The figure shows three views and two pictorial views of one solid part (mm, origin at its lowest corner). Answer the questions. A direction names the side the tool comes from. Round coordinates to 2 decimals unless told otherwise and drop trailing zeros. Order: outer loops, then holes, each group sorted by start corner. A loop starts at its lowest first (then second) coordinate and runs counter-clockwise, first axis right, second up. Notation, with made-up numbers: (54.25, 15) -> (87.25, 15) arc R24 ccw to (87.25, 48) -> close; hole circle Ø9 at (79, 0.5). An arc over 180 degrees is marked (long way). Answer as a JSON object with one key per item and string values. Group by question number.
Item 1: The mould has two halves that part along Z. Classify the marked faces 3, 4 and 5: pulls with the +Z half, pulls with the -Z half, needs draft (parallel to the pull), parting line crosses it, or undercut.
Item 2: Section B-B, the plane y = 7.5 is taken. Write down the section's boundary in (x, z) (1 decimal).
Item 3: Given P1, Ø4, axis at x = 38, y = 9.5, coming from the -Z side; P2, Ø10, axis at y = 6, z = 99.5, coming from the +X side (1 decimal); P3, Ø10, axis at x = 16.5, z = 29, coming from the +Y side (1 decimal), each flat-ended and moving along its own axis, determine where each tip first touches the part or whether it passes through.
Item 4: Section A-A, the plane y = 27 is taken. Write down the section's boundary in (x, z), plus the area to 3 significant figures.
Item 5: Section C-C, the plane z = 10.5 is taken. Write down the section's boundary in (x, y) (1 decimal), plus the area to 3 significant figures.
Item 6: Consider probe 1 along Z at (x, y) = (55, 29) (1 decimal); probe 2 along X at (y, z) = (30.5, 67) (1 decimal); probe 3 along Y at (x, z) = (105.5, 46) (1 decimal). Determine where each line is inside the solid, lowest interval first. Write a range as from..to.
Item 7: For the marked faces 1 and 2, determine the directions among +Z, -Z, +X, -X, +Y, -Y from which every point of the face is accessible in a straight line to the end or side of a thin tool.
Item 8: Section D-D, the plane x = 98 is taken. Write down the section's boundary in (y, z) (1 decimal).
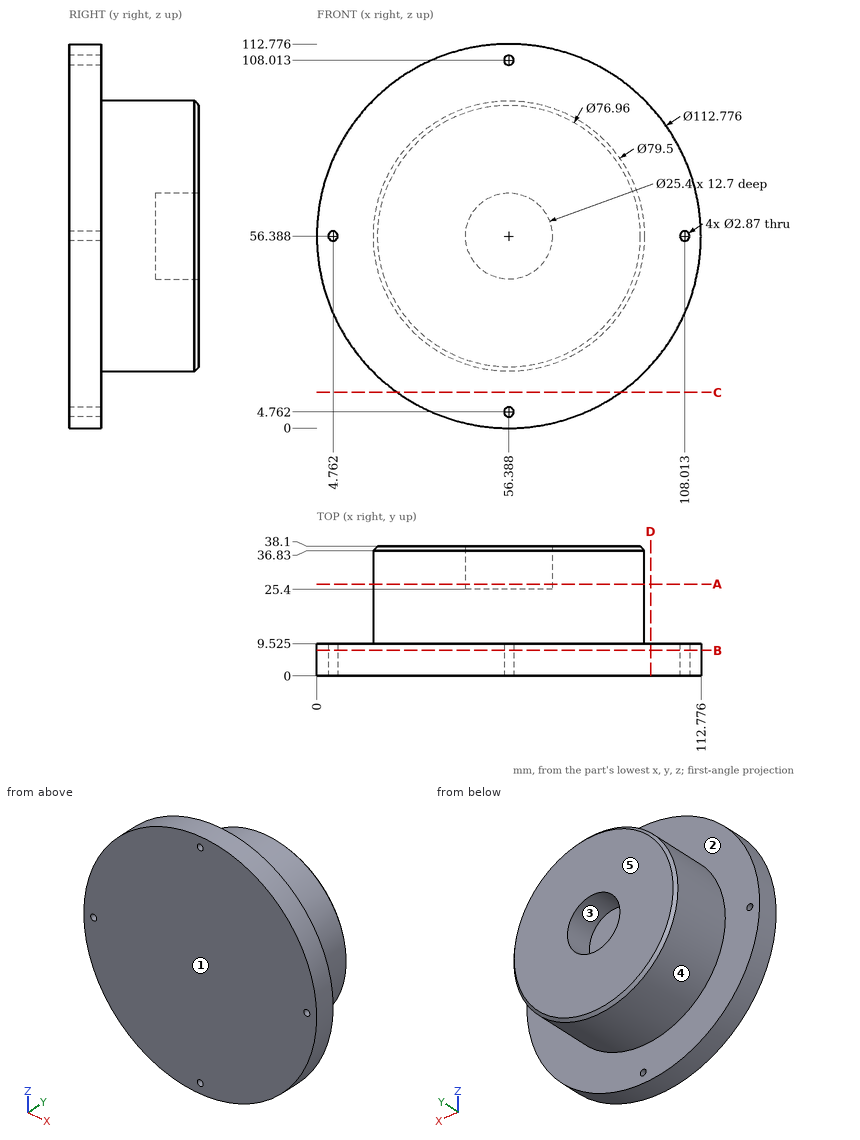
Values found:
{
 "1": {"face 3": "undercut", "face 4": "parting line crosses it", "face 5": "needs draft"},
 "2": {"outline": "circle Ø112.8 at (56.4, 56.4); hole circle Ø2.9 at (4.8, 56.4); hole circle Ø2.9 at (56.4, 4.8); hole circle Ø2.9 at (56.4, 108); hole circle Ø2.9 at (108, 56.4)"},
 "3": {"P1": "z = 2.43", "P2": "x = 97.9", "P3": "y = 9.5"},
 "4": {"outline": "circle Ø79.5 at (56.39, 56.39); hole circle Ø25.4 at (56.39, 56.39)", "area": "4,460 mm2"},
 "5": {"outline": "(23.6, 0) -> (89.2, 0) -> (89.2, 9.5) -> (23.6, 9.5) -> close", "area": "624 mm2"},
 "6": {"probe 1": "16.7..43.8, 69..96.1", "probe 2": "18.1..49.4, 63.4..94.7", "probe 3": "0..9.5"},
 "7": {"face 1": "+Z, -Z, +X, -X, -Y", "face 2": "+Y"},
 "8": {"outline": "(0, 18.3) -> (9.5, 18.3) -> (9.5, 94.4) -> (0, 94.4) -> close"}
}
